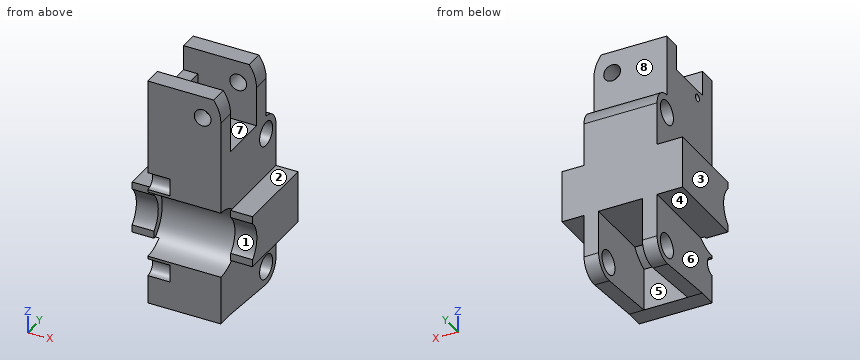
Autodesk Inventor part; units mm, degrees
ref_plane "YZ Plane" through (0, 0, 0) normal (1, 0, 0) x (0, 1, 0)
ref_plane "XZ Plane" through (0, 0, 0) normal (0, 1, 0) x (-1, 0, 0)
ref_plane "XY Plane" through (0, 0, 0) normal (0, 0, 1) x (1, 0, 0)
sketch "スケッチ1" plane through (0, 0, 0) normal (1, 0, 0) x (0, 1, 0)
  circle A0 centre (0, 0) radius 4.575
  circle A1 centre (0, 0) radius 3.575
  line L0 (0, 0) -> (0, 6)
  line L1 (0, 6) -> (0, -6)
  line L2 (0, 0) -> (11.5, 0)
  line L3 (11.5, 0) -> (11.5, 9.5)
  line L4 (11.5, 9.5) -> (11.5, -9.5)
  circle A2 centre (11.5, 9.5) radius 1.65
  circle A3 centre (11.5, -9.5) radius 1.65
  line L5 (0, 0) -> (0, 11.25)
  line L6 (0, 11.25) -> (0, -11.25)
  line L7 (-2.5, -11.25) -> (2.5, -11.25)
  line L8 (2.5, -11.25) -> (2.5, 11.25)
  line L9 (2.5, 11.25) -> (-2.5, 11.25)
  line L10 (-2.5, 11.25) -> (-2.5, -11.25)
  line L11 (-2.5, -11.25) -> (2.5, 11.25) construction
  line L12 (2.5, -11.25) -> (-2.5, 11.25) construction
  circle A4 centre (11.5, 9.5) radius 2.5
  circle A5 centre (11.5, -9.5) radius 2.5
  line L13 (2.5, 11.25) -> (11.2899, 11.9912)
  line L14 (2.5, -11.25) -> (11.2899, -11.9912)
  line L15 (14, 9.5) -> (14, -9.5)
  line L16 (0, -3.575) -> (14, -3.575)
  line L17 (0, 3.575) -> (14, 3.575)
  circle A6 centre (0, 0) radius 6
  line L18 (0, 0) -> (0, 6.15)
  line L19 (0, 6.15) -> (0, -6.15)
  circle A7 centre (0, 6.15) radius 1.25
  circle A8 centre (0, -6.15) radius 1.25
  line L20 (0, 11.25) -> (11.5, 11.25)
  line L21 (11.5, 11.25) -> (11.5, 12)
  line L22 (11.5, 12) -> (0, 12)
  line L23 (0, 12) -> (0, 11.25)
  point P0 (0, 4.575)
  point P1 (0, -4.575)
  point P2 (2.5, 3.575)
  point P3 (2.5, 2.5555)
  point P4 (2.5, -2.5555)
  point P5 (2.5, -3.575)
  point P6 (0, 7.4)
  point P7 (0, 4.9)
  point P8 (0, -4.9)
  point P9 (0, -7.4)
  point P10 (2.5, 5.4544)
  point P11 (2.5, -5.4544)
  point P12 (4.8186, 3.575)
  point P13 (4.8186, -3.575)
  point P14 (2.8548, 3.575)
  point P15 (2.8548, -3.575)
  dimension "d0" = 9.15
  dimension "d1" = 7.15
  dimension "d2" = 6
  dimension "d3" = 12
  dimension "d6" = 11.5
  dimension "d7" = 9.5
  dimension "d8" = 19
  dimension "d9" = 3.3
  dimension "d10" = 3.3
  dimension "d11" = 11.25
  dimension "d12" = 22.5
  dimension "d13" = 5
  dimension "d14" = 5
  dimension "d15" = 5
  dimension "d28" = 12
  dimension "d29" = 6.15
  dimension "d30" = 12.3
  dimension "d31" = 2.5
  dimension "d32" = 2.5
  dimension "d89" = 11.5
extrude "押し出し7" add sketch "スケッチ1" along normal blind 2 contours L2 A6 L16 A0 | A0 L17 A6 L2 | A0 L8 A6 L17 | L16 A6 L8 A0 | A6 L17 L3 L2 | L2 L4 L16 A6 | A0 L0 A7 A6 L8 | A6 L8 L20 A4 L3 L17 | L8 A6 A8 L1 A0 | L16 L4 A5 L14 L8 A6 | L3 L17 L15 L16 L4 | A6 A7 L5 L9 L8 | L3 A4 L15 L17 | L8 L7 L6 A8 A6 | L16 L15 A5 L4 | L13 A4 L20 | A4 L20 L21 | A5 | A4 L21 L20
extrude "押し出し8" add sketch "スケッチ1" along normal blind 10 contours L2 A6 L16 A0 | A0 L17 A6 L2 | A0 L8 A6 L17 | L16 A6 L8 A0 | A6 L17 L3 L2 | L2 L4 L16 A6 | A0 L0 A7 A6 L8 | L8 A6 A8 L1 A0 | L3 L17 L15 L16 L4 | A6 A7 L5 L9 L8 | L8 L7 L6 A8 A6 | L0 A6 A7 | A6 L5 A7 | A8 A6 L1 | A8 L6 A6 picked at (0.2292, 5.6392) picked at (0.3961, 6.4211) picked at (0.2292, -5.6392) picked at (0.3961, -6.4211)
sketch "スケッチ6" plane through (10, 0, 0) normal (1, 0, 0) x (0, 0, -1)
  line L0 (0, 0) -> (-6.15, 0)
  line L1 (-6.15, 0) -> (6.15, 0)
  circle A0 centre (-6.15, 0) radius 1.25
  circle A1 centre (6.15, 0) radius 1.25
  line L2 (-11.25, 2.5) -> (11.25, 2.5)
  line L3 (11.25, 2.5) -> (11.25, -2.5)
  line L4 (11.25, -2.5) -> (-11.25, -2.5)
  line L5 (-11.25, -2.5) -> (-11.25, 2.5)
  line L6 (-11.25, 2.5) -> (11.25, -2.5) construction
  line L7 (11.25, 2.5) -> (-11.25, -2.5) construction
  line L8 (0, 0) -> (0, 11.5)
  line L9 (0, 11.5) -> (-9.5, 11.5)
  line L10 (-9.5, 11.5) -> (9.5, 11.5)
  circle A2 centre (-9.5, 11.5) radius 1.65
  circle A3 centre (-9.5, 11.5) radius 2.5
  circle A4 centre (9.5, 11.5) radius 1.65
  circle A5 centre (9.5, 11.5) radius 2.5
  circle A6 centre (0, 0) radius 6
  circle A7 centre (0, 0) radius 4.575
  arc A8 (11.9912, 11.2899) -> (9.5, 14) centre (9.5, 11.5) ccw
  line L11 (11.25, 2.5) -> (11.9912, 11.2899)
  line L12 (-11.9912, 11.2899) -> (-11.25, 2.5)
  line L13 (-11.25, 2.5) -> (-11.9912, 11.2899)
  line L14 (9.5, 14) -> (-9.5, 14)
  arc A9 (-9.5, 14) -> (-11.9912, 11.2899) centre (-9.5, 11.5) ccw
  line L15 (-9.5, 14) -> (9.5, 14)
  circle A10 centre (0, 0) radius 3.575
  line L16 (-3.575, 14) -> (-3.575, 4.8186)
  line L17 (3.575, -14) -> (-3.575, -14)
  line L18 (-3.575, -14) -> (-3.575, 14)
  line L19 (-3.575, 14) -> (3.575, 14)
  line L20 (3.575, 14) -> (3.575, -14)
  line L21 (3.575, -14) -> (-3.575, 14) construction
  line L22 (-3.575, -14) -> (3.575, 14) construction
  line L23 (-11.25, 0) -> (-12.0089, 0)
  line L24 (-12.0089, 0) -> (-12.0089, 11.5)
  line L25 (-12.0089, 11.5) -> (-11.25, 11.5)
  line L26 (-11.25, 11.5) -> (-11.25, 0)
  line L27 (-12.0089, 0) -> (-12.0089, 5.75)
  line L28 (-20.4427, 2.45) -> (-3.575, 2.45)
  line L29 (-3.575, 2.45) -> (-3.575, 9.05)
  line L30 (-3.575, 9.05) -> (-20.4427, 9.05)
  line L31 (-20.4427, 9.05) -> (-20.4427, 2.45)
  line L32 (-20.4427, 2.45) -> (-3.575, 9.05) construction
  line L33 (-3.575, 2.45) -> (-20.4427, 9.05) construction
  line L34 (-3.575, 0) -> (-20.4427, 0)
  line L35 (-20.4427, 0) -> (-20.4427, 11.5)
  line L36 (-20.4427, 11.5) -> (-3.575, 11.5)
  line L37 (-3.575, 11.5) -> (-3.575, 0)
  line L38 (-3.575, 0) -> (-20.4427, 11.5) construction
  line L39 (-20.4427, 0) -> (-3.575, 11.5) construction
  point P0 (-5.4544, 2.5)
  point P1 (5.4544, 2.5)
  point P2 (7, 11.5)
  point P3 (-7, 11.5)
  point P4 (-3.575, 11.5)
  point P5 (-3.575, 4.8186)
  point P6 (-3.575, 2.5)
  point P7 (-2.5555, 2.5)
  point P8 (2.5555, 2.5)
  point P9 (3.575, 2.5)
  point P10 (3.575, 11.5)
  point P11 (-9.9975, 9.05)
  point P12 (-9.0025, 9.05)
  point P13 (-12, 11.5)
  point P14 (-12.0089, 9.05)
  point P15 (-12.0089, 2.45)
  dimension "d69" = 12
  dimension "d56" = 6.15
  dimension "d57" = 12.3
  dimension "d58" = 2.5
  dimension "d59" = 2.5
  dimension "d62" = 11.5
  dimension "d63" = 9.5
  dimension "d64" = 19
  dimension "d65" = 3.3
  dimension "d66" = 5
  dimension "d67" = 3.3
  dimension "d68" = 5
  dimension "d70" = 9.15
  dimension "d79" = 7.15
  dimension "d90" = 5.75
  dimension "d91" = 6.6
extrude "押し出し9" add sketch "スケッチ6" against normal blind 2 contours A6 L20 L10 A5 L11 L2 | A6 L8 L10 L20 | A6 L16 L9 L8 | L2 L26 L30 A3 L16 A6 | L20 L14 A5 L10 | L10 L9 L16 L14 L20 | L12 L30 L26 | L30 A3 L9 L16 | A5 | L9 A3 L14 L16 | L12 A3 L26 L30 | L26 A3 L30 | L30 A3 L26 L36 A2 L9 | A3 L30 | L9 A2 L36 L25 A3 | A3 L25 L26
extrude "押し出し10" add sketch "スケッチ1" against normal blind 0.5 contours L2 A6 L16 A0 | A0 L17 A6 L2 | A6 L17 L3 L2 | L2 L4 L16 A6 | L3 L17 L15 L16 L4
sketch "スケッチ7" plane through (-0.5, 0, 0) normal (-1, 0, 0) x (0, 0, 1)
  circle A0 centre (0, 0) radius 3.575
  line L0 (-9.5, 14) -> (9.5, 14)
  line L1 (-3.575, 14) -> (3.575, 14)
  circle A1 centre (0, 0) radius 4.575
  line L2 (-11.25, 0) -> (-11.25, 2.5)
  line L3 (11.25, -2.5) -> (-11.25, -2.5)
  line L4 (-11.25, -2.5) -> (-11.25, 2.5)
  line L5 (-11.25, 2.5) -> (11.25, 2.5)
  line L6 (11.25, 2.5) -> (11.25, -2.5)
  line L7 (11.25, -2.5) -> (-11.25, 2.5) construction
  line L8 (-11.25, -2.5) -> (11.25, 2.5) construction
  line L9 (-3.575, 14) -> (-3.575, 0)
  line L10 (3.575, 14) -> (3.575, 0)
  point P0 (-3.575, 2.5)
  point P1 (-2.5555, 2.5)
  point P2 (2.5555, 2.5)
  point P3 (3.575, 2.5)
  dimension "d75" = 7.15
  dimension "d76" = 5
extrude "押し出し11" add sketch "スケッチ7" along normal blind 3 contours A0 L5 L9 A1 L10 | A1 L9 L0 L10
extrude "押し出し12" add sketch "スケッチ6" along normal blind 3 contours L2 L18 A7 L8 A10 | A10 L8 A7 L20 L2 | A7 L8 A6 L20 | A7 L18 A6 L8 | A6 L8 L10 L20 | A6 L16 L9 L8 | L10 L9 L16 L14 L20
hole "穴1" at (0, 0, -6.15) at (0, 0, 6.15) direction (1, 0, 0) diameter 2.4 depth 3
sketch "スケッチ8" plane through (0, 11.2899, 11.9912) normal (0, -0.084, 0.9965) x (1, 0, 0)
  point P0 (0, -12.2575)
extrude "押し出し13" add sketch "スケッチ6" against normal blind 10 contours L2 L26 L30 A3 L16 A6 | L28 L24 L30 L12 L5 | L5 L23 L24 L28 | L12 L30 L26 | L24 L34 L35 L28 | L30 A3 L9 L16 | L9 A3 L14 L16 | L30 L24 L25 A3 L12 | L12 A3 L26 L30 | L26 A3 L30 | L30 A3 L26 L36 A2 L9 | L9 A2 L36 L25 A3 | A3 L25 L26 | L30 L35 L36 L24
sketch "スケッチ9" plane through (10, 11.5, 20.4427) normal (0, 1, 0) x (1, 0, 0)
  line L0 (-10, 8.4427) -> (0, 8.4427)
  line L1 (0, 8.4427) -> (-5, 8.4427)
  line L2 (0, 0) -> (-10, 0)
  line L3 (-5, 0) -> (-5, 3)
  circle A0 centre (-5, 3) radius 1.15
  circle A1 centre (-5, 3) radius 5
  line L4 (0, 8.4427) -> (0, 0)
  line L5 (0, -2.4427) -> (-10, -2.4427)
  line L6 (-10, -2.4427) -> (-10, 8.4427)
  line L7 (-10, 8.4427) -> (0, 8.4427)
  line L8 (0, 8.4427) -> (0, -2.4427)
  line L9 (0, -2.4427) -> (-10, 8.4427) construction
  line L10 (-10, -2.4427) -> (0, 8.4427) construction
  line L11 (0, 0) -> (-10, 0)
  line L12 (-10, 0) -> (0, 0)
  line L13 (-10, 0) -> (-10, 8.4427)
  line L14 (-10, 3) -> (-7, 3)
  circle A2 centre (-7, 3) radius 1.15
  line L15 (-5, 3) -> (-2.5, 3)
  circle A3 centre (-2.5, 3) radius 1.15
  point P0 (-10, 20.4427)
  point P1 (0, 3)
  point P2 (-1, 0)
  point P3 (-9, 0)
  dimension "d94" = 3
  dimension "d95" = 2.3
  dimension "d98" = 3
  dimension "d99" = 2.3
  dimension "d100" = 2.3
extrude "押し出し14" cut sketch "スケッチ9" against normal blind 11.5 contours A3 | L4 L2 A1
sketch "スケッチ10" plane through (10, 2.45, 12.0089) normal (0, 0, 1) x (1, 0, 0)
  point P0 (-10, -2.45)
sketch "スケッチ11" plane through (10, 2.45, 12.0089) normal (0, 0, 1) x (1, 0, 0)
  line L0 (-10, 0) -> (-10, 6.6)
  line L1 (0, 0) -> (-10, 0)
  line L2 (-10, 6.6) -> (-7.6825, 6.6)
  line L3 (-7.6825, 6.6) -> (-7.6825, 0)
  line L4 (-7.6825, 0) -> (-10, 0)
  line L5 (-10, 0) -> (-10, 6.6)
  line L6 (-8, 0.05) -> (-8, 8.8399)
  line L7 (-10, 6.6) -> (-8, 6.6)
  line L8 (-8, 6.6) -> (-8, 0.05)
  line L9 (-8, 0.05) -> (-10, 0.05)
  line L10 (-10, 0.05) -> (-10, 6.6)
  line L11 (-10, 0.05) -> (-8, 0.05)
  line L12 (-8, 0.05) -> (-8, 0)
  line L13 (-8, 0) -> (-10, 0)
  line L14 (-10, 0) -> (-10, 0.05)
  point P0 (-10, -2.45)
extrude "押し出し15" add sketch "スケッチ11" along normal blind 5 contours L0 L9 L12 L1 | L0 L2 L6 L9
sketch "スケッチ12" plane through (2, 2.45, 12.0089) normal (1, 0, 0) x (0, 0, -1)
  line L0 (0, 0) -> (-5, 0)
  line L1 (-8.4339, 6.6) -> (-8.4339, 9.05)
  line L2 (0, 0) -> (-8.4339, 0)
  line L3 (-8.4339, 0) -> (-8.4339, 9.05)
  line L4 (-8.4339, 9.05) -> (0, 9.05)
  line L5 (0, 9.05) -> (0, 0)
  line L6 (-8.4339, 0) -> (-5, 0)
  line L7 (-8.4339, 0) -> (-3.9339, 0)
  line L8 (-3.9339, 0) -> (-3.9339, 2.6858)
  line L9 (-3.9339, 2.6858) -> (-8.4339, 2.6858)
  line L10 (-8.4339, 2.6858) -> (-8.4339, 0)
  line L11 (-3.9339, 0) -> (-3.9339, 3.3)
  line L12 (-3.9339, 3.3) -> (-3.9339, 1.3)
  point P0 (12.0089, -2.45)
  dimension "d103" = 4.5
  dimension "d104" = 3.3
  dimension "d105" = 2
hole "穴2" at (2, 3.75, 15.9427) direction (-1, 0, 0) diameter 1 depth 8
properties part number "ikafly5.0d"
Source: CAD feature listing. Evaluate the final solid. Frame: model axes, mm. Face numbers are marked on the shaded views. A direction names the side the tool comes from. Coordinates: 2 decimals unless noted, no trailing zeros. Loops run counter-clockwise (first coordinate to the right, second up) from the corner with the lowest first, then second, coordinate; pieces in that order, holes last. Notation, with made-up numbers: M 87,34.5 L 103,34.5 A18 ccw 103,61.5 Z; hole C 28.5,-14.75 d7. An arc over 180 degrees is marked long. Use CSV: the item, a comma, the result in double quotes.
(1) Cut plane C-C on z = 0. Return loops of the section in (x, y) (3 decimals), and give its area (3 significant figures).
Answers follow:
outline,"M -3.5,3.575 L -0.5,3.575 L -0.5,4.575 L 10,4.575 L 10,3.575 L 13,3.575 L 13,14 L -3.5,14 Z"
area,"162 mm²"
(2) Contact query for flat-ended pins moving along their axis: pin 1 (5 mm diameter, centred on x = 3, z = -0.5, fed in from -Y); pin 2 (1.2 mm diameter, centred on x = 7, y = 1.5, fed in from -Z); pin 3 (1.8 mm diameter, centred on x = -2, y = 5.5, fed in from -Z) (3 decimals). Output: stop coordinate, or through.
Answers follow:
pin 1,"y = 3.45"
pin 2,"z = -11.25"
pin 3,"z = -3.575"
(3) Draft query along Z for the marked faces 1, 2, 3 and 4. Return one class per face: pulls with the +Z half, pulls with the -Z half, needs draft (parallel to the pull), parting line crosses it, or undercut.
Answers follow:
face 1,"undercut"
face 2,"pulls with the +Z half"
face 3,"needs draft"
face 4,"pulls with the -Z half"
(4) Cut plane A-A on x = 7.5. Give the number of separate pieces and of enclosed holes in the cut face, and give its area (3 significant figures).
Answers follow:
separate pieces,"3"
enclosed holes,"2"
area,"227 mm²"
(5) Reachability of the marked faces 5, 6, 7 and 8 from +Z, -Z, +X, -X, +Y, -Y: full face, straight path, thin tool, end or side. Return the list, or none.
Answers follow:
face 5,"-Z, +Y"
face 6,"-Z, -X, +Y, -Y"
face 7,"+Z, +X"
face 8,"+Z, +X, -X, +Y"
(6) Cut plane D-D on y = 7.5. Return loops of the section in (x, z) (3 decimals), and give its area (3 significant figures).
Answers follow:
outline,"M -3.5,-3.575 L 0,-3.575 L 0,-11.672 L 2,-11.672 L 2,-3.575 L 8,-3.575 L 8,-11.672 L 10,-11.672 L 10,-3.575 L 13,-3.575 L 13,3.575 L 10,3.575 L 10,12.009 L 2,12.009 L 2,17.009 L 0,17.009 L 0,3.575 L -3.5,3.575 Z"
area,"245 mm²"
(7) Line query: line 1 (Y direction, x = 0.75, z = 19); line 2 (Z direction, x = 7.5, y = 9.8) (3 decimals); line 3 (Y direction, x = 1.25, z = -9.5). Output: solid intervals per line, ascending. Write a range as [from, to].
Answers follow:
line 1,"[0, 2.45], [9.05, 11.5]"
line 2,"[-3.575, 16.293], [18.593, 20.443]"
line 3,"[0, 9.85], [13.15, 14]"
